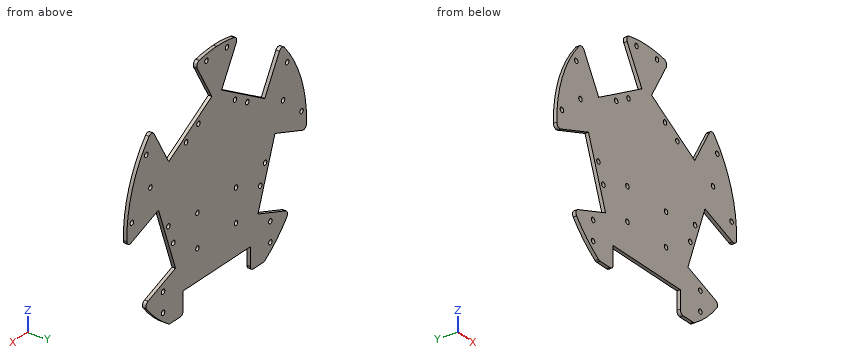
```python
from build123d import *

# Parameters (mm, degrees)
CUTOFF_PROFILE_DEPTH = 2.5
FLANGED_HOLES_D      = 3.4
EXCESS_START         = -10
EXCESS_CUT_DEPTH     = 10
M3_CLEARANCE_HOLE1_D = 3.4
FILLET1_R            = 3
CUT_EXTRUDE2_START   = -2.5
CUT_EXTRUDE2_DEPTH   = 2.5
FILLET2_R            = 3
M3_CLEARANCE_HOLE2_D = 3.4


with BuildPart() as part:
    # Sketch1 → cutoff profile (new body)
    with BuildSketch(Plane(origin=(0, 0, 0), x_dir=(1, 0, 0), z_dir=(0, 1, 0))):
        with BuildLine():
            Line((-33, 83.194050268), (-33, 59.194050268))
            Line((-33, 59.194050268), (33, 59.194050268))
            Line((33, 59.194050268), (33, 83.194050268))
            ThreePointArc((33, 83.194050268), (54.947257978, 70.647355511), (72.510522323, 52.464027222))
            Line((72.510522323, 52.464027222), (40.560973217, 40.835342349))
            Line((40.560973217, 40.835342349), (57.31996024, -5.209596069))
            Line((57.31996024, -5.209596069), (89.269509346, 6.419088804))
            ThreePointArc((89.269509346, 6.419088804), (84.10248956, -30.610802828), (64.258300826, -62.298641839))
            Line((64.258300826, -62.298641839), (47.258300826, -32.85377811))
            Line((47.258300826, -32.85377811), (4.823056041, -57.35377811))
            Line((4.823056041, -57.35377811), (21.823056041, -86.798641839))
            ThreePointArc((21.823056041, -86.798641839), (0, -89.5), (-21.823056041, -86.798641839))
            Line((-21.823056041, -86.798641839), (-4.823056041, -57.35377811))
            Line((-4.823056041, -57.35377811), (-47.258300826, -32.85377811))
            Line((-47.258300826, -32.85377811), (-64.258300826, -62.298641839))
            ThreePointArc((-64.258300826, -62.298641839), (-84.10248956, -30.610802828), (-89.269509346, 6.419088804))
            Line((-89.269509346, 6.419088804), (-57.31996024, -5.209596069))
            Line((-57.31996024, -5.209596069), (-40.560973217, 40.835342349))
            Line((-40.560973217, 40.835342349), (-72.510522323, 52.464027222))
            ThreePointArc((-72.510522323, 52.464027222), (-54.947257978, 70.647355511), (-33, 83.194050268))
        make_face()
    extrude(amount=CUTOFF_PROFILE_DEPTH)

    # flanged holes (through all)
    with Locations(Plane(origin=(0, 2.5, 0), x_dir=(1, 0, 0), z_dir=(0, 1, 0))):
        with Locations((52.8, 65), (-17.978500607, -45.139676495), (-47.575837248, 9.866944221), (-30.10285626, -38.139676495), (-42.787555242, 23.022640912), (17.978500607, -45.139676495), (30.10285626, -38.139676495), (47.575837248, 9.866944221), (42.787555242, 23.022640912), (65.268611951, -23.755831982), (-65.268611951, -23.755831982), (-52.8, 51), (52.8, 51), (-52.8, 65)):
            Hole(FLANGED_HOLES_D / 2)

    # Sketch5 → excess cut (cut)
    with BuildSketch(Plane(origin=(0, 2.5, 0), x_dir=(1, 0, 0), z_dir=(0, 1, 0)).offset(EXCESS_START)):
        with BuildLine():
            ThreePointArc((21.302960858, -85.897810558), (10.730651555, -87.847043873), (0, -88.5))
            ThreePointArc((0, -88.5), (-10.730651555, -87.847043873), (-21.302960858, -85.897810558))
            Line((-21.302960858, -85.897810558), (-21.823056041, -86.798641839))
            ThreePointArc((-21.823056041, -86.798641839), (0, -89.5), (21.823056041, -86.798641839))
            Line((21.823056041, -86.798641839), (21.302960858, -85.897810558))
        make_face()
        with BuildLine():
            ThreePointArc((-64.258300826, -62.298641839), (0, 89.5), (64.258300826, -62.298641839))
            Line((64.258300826, -62.298641839), (63.738205644, -61.397810558))
            ThreePointArc((63.738205644, -61.397810558), (0, 88.5), (-63.738205644, -61.397810558))
            Line((-63.738205644, -61.397810558), (-64.258300826, -62.298641839))
        make_face()
    extrude(amount=EXCESS_CUT_DEPTH, mode=Mode.SUBTRACT)

    # M3 Clearance Hole1 (through all)
    with Locations(Plane(origin=(0, 2.5, 0), x_dir=(1, 0, 0), z_dir=(0, 1, 0))):
        with Locations((19, 37.217294159), (-19, 13.617294159), (-19, 37.217294159), (19, 13.617294159)):
            Hole(M3_CLEARANCE_HOLE1_D / 2)

    # Fillet1
    fillet1_edges = [part.edges().sort_by_distance(p)[0] for p in [
        (-21.302960858, 1.25, 85.897810558),
        (21.302960858, 1.25, 85.897810558),
        (-63.738205644, 1.25, 61.397810558),
        (-88.292050136, 1.25, -6.063322746),
        (88.292050136, 1.25, -6.063322746),
        (33, 1.25, -82.117294159),
        (-33, 1.25, -82.117294159),
        (-71.533063113, 1.25, -52.108261165),
        (71.533063113, 1.25, -52.108261165),
        (63.738205644, 1.25, 61.397810558),
    ]]
    fillet(fillet1_edges, radius=FILLET1_R)

    # Sketch9 → Cut-Extrude2 (cut)
    with BuildSketch(Plane(origin=(0, 2.5, 0), x_dir=(1, 0, 0), z_dir=(0, 1, 0)).offset(CUT_EXTRUDE2_START)):
        with BuildLine():
            ThreePointArc((-37.263157895, 80.27270435), (-36.646789817, 80.481043276), (-36, 80.551595728))
            ThreePointArc((-36, 80.551595728), (-33.878679656, 79.672916072), (-33, 77.551595728))
            Line((-33, 77.551595728), (-33, 75.201595728))
            Line((-33, 75.201595728), (33, 75.201595728))
            Line((33, 75.201595728), (33, 77.551595728))
            ThreePointArc((33, 77.551595728), (34.385917239, 80.08037742), (37.263157895, 80.27270435))
            ThreePointArc((37.263157895, 80.27270435), (42.037122726, 77.878946532), (46.658011101, 75.201595728))
            Line((46.658011101, 75.201595728), (56.845139831, 75.201595728))
            Line((56.845139831, 75.201595728), (56.845139831, 82.959992601))
            Line((56.845139831, 82.959992601), (-46.658011101, 82.959992601))
            Line((-46.658011101, 82.959992601), (-46.658011101, 75.201595728))
            ThreePointArc((-46.658011101, 75.201595728), (-42.037122726, 77.878946532), (-37.263157895, 80.27270435))
        make_face()
        with BuildLine():
            Line((-36, 75.201595728), (-36, 80.551595728))
            ThreePointArc((-36, 80.551595728), (-36.646789817, 80.481043276), (-37.263157895, 80.27270435))
            ThreePointArc((-37.263157895, 80.27270435), (-42.037122726, 77.878946532), (-46.658011101, 75.201595728))
            Line((-46.658011101, 75.201595728), (-36, 75.201595728))
        make_face()
        with BuildLine():
            ThreePointArc((-33, 77.551595728), (-33.878679656, 79.672916072), (-36, 80.551595728))
            Line((-36, 80.551595728), (-36, 75.201595728))
            Line((-36, 75.201595728), (-33, 75.201595728))
            Line((-33, 75.201595728), (-33, 77.551595728))
        make_face()
        with BuildLine():
            Line((33, 77.551595728), (33, 75.201595728))
            Line((33, 75.201595728), (46.658011101, 75.201595728))
            ThreePointArc((46.658011101, 75.201595728), (42.037122726, 77.878946532), (37.263157895, 80.27270435))
            ThreePointArc((37.263157895, 80.27270435), (34.385917239, 80.08037742), (33, 77.551595728))
        make_face()
    extrude(amount=CUT_EXTRUDE2_DEPTH, mode=Mode.SUBTRACT)

    # Fillet2
    fillet2_edges = [part.edges().sort_by_distance(p)[0] for p in [
        (-33, 1.25, -75.201595728),
        (-46.658011101, 1.25, -75.201595728),
        (33, 1.25, -75.201595728),
        (46.658011101, 1.25, -75.201595728),
    ]]
    fillet(fillet2_edges, radius=FILLET2_R)

    # M3 Clearance Hole2 (through all)
    with Locations(Plane(origin=(0, 2.5, 0), x_dir=(1, 0, 0), z_dir=(0, 1, 0))):
        with Locations((83.517603132, -8.443110213), (-69.405322414, -47.216282822), (-83.517603132, -8.443110213), (10.101112813, -83.386243549), (-10.101112813, -83.386243549), (69.405322414, -47.216282822)):
            Hole(M3_CLEARANCE_HOLE2_D / 2)


solid = part.part
```
For this review, take the finished solid that the model builds, in its own axes (mm). Coordinates: 2 decimals unless noted, no trailing zeros. Write each loop counter-clockwise with the first axis right and the second up, starting at its lowest first coordinate (ties: lowest second). Pieces come first, ordered by that corner, then holes. Notation, with made-up numbers: (89.25, 72) -> (95.25, 72) arc R35 cw to (95.25, 105) -> close; hole circle Ø5 at (-11, 19.5). An arc over 180 degrees is marked (long way). Put each result on its own line as item: value.
Q1. Clearance check with flat-ended pins moving along their axes: pin 1 Ø2.5 at (x, z) = (47.58, -9.87) entering from +Y; pin 2 Ø1.5 at (y, z) = (1, 5.5) entering from +X; pin 3 Ø0.8 at (y, z) = (1.5, -63.5) entering from -X; pin 4 Ø1.5 at (x, y) = (69.5, 2) entering from -Z. State where each tip first meets the part, or that it passes through.
From the geometry:
pin 1: passes through
pin 2: stops at x = 88.37
pin 3: stops at x = -62.05
pin 4: stops at z = -55.73
Q2. Take a section at B-B, the plane x = -23. State the section outline as (y, z) points, then the cut area to 3 significant figures.
From the geometry:
outline: (0, -59.19) -> (2.5, -59.19) -> (2.5, 46.86) -> (0, 46.86) -> close
area: 265 mm2
Q3. Take a section at A-A, the plane y = 0.9. Count the separate pieces of the cut face and the enclosed holes in it, then the cut area to 3 significant figures.
From the geometry:
separate pieces: 1
enclosed holes: 24
area: 15,500 mm2
Q4. Wall thickness on L1, parallel to X at y = 0.7, z = 54; L2, parallel to X at y = 0.85, z = -51; L3, parallel to Z at x = 18.5, y = 2.3: over which ranges is each line inside the solid? List them lowest first.
From the geometry:
L1: x = -70.12 to -59.47, -10.63 to 10.63, 59.47 to 70.12
L2: x = -68.28 to -54.5, -51.1 to 51.1, 54.5 to 68.28
L3: z = -59.19 to -38.84, -35.59 to -15.24, -11.99 to 43.52, 46.76 to 49.46, 81.04 to 86.23
